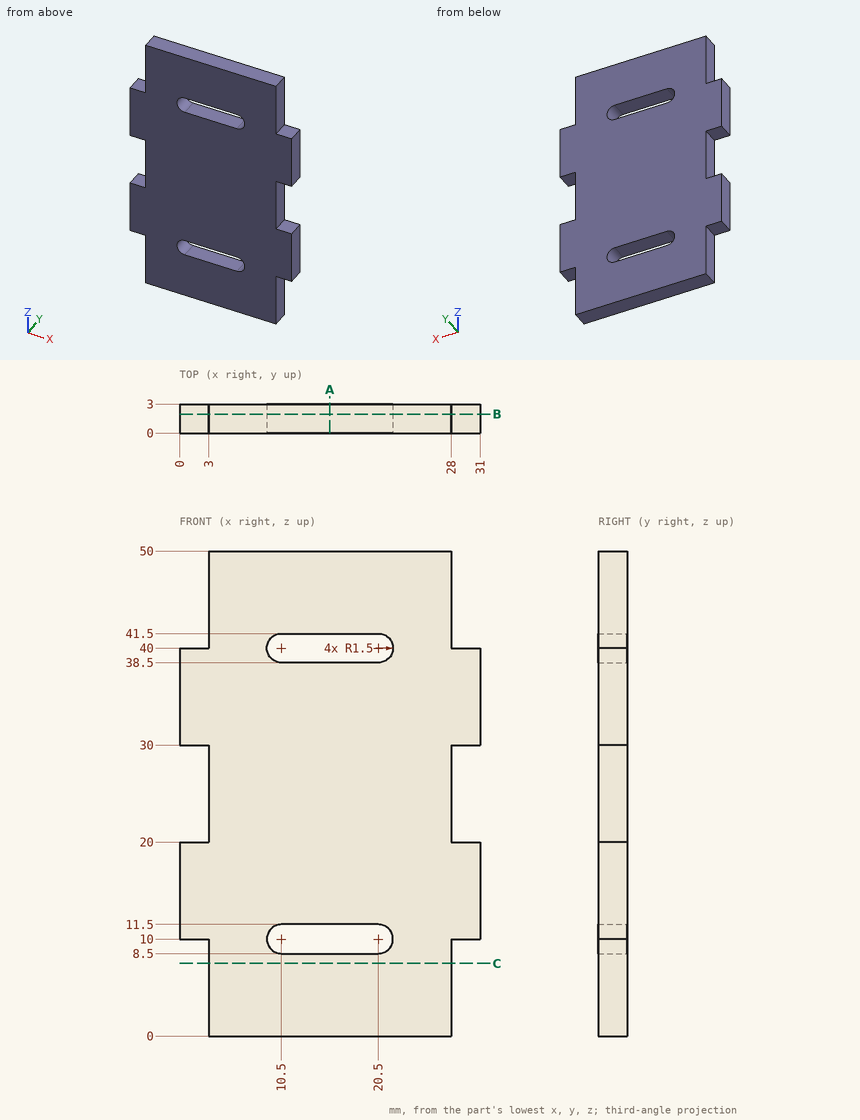
Print and shaded views of the part. All mm, measured from the part's lowest x, y and z. Give positions to 0.01 mm unless a question says otherwise; leave off trailing zeros. Loops run counter-clockwise (first coordinate to the right, second up) from the corner with the lowest first, then second, coordinate; pieces in that order, holes last. Notation, with made-up numbers: (20, -33.5) -> (37, -33.5) arc R7 ccw to (37, -22.5) -> close; hole circle Ø7 at (41, -11.75). An arc over 180 degrees is marked (long way). Use CSV: the item, a comma, the result in double quotes. Start each with the question number.
1) Wall check: line 1 (Z direction, x = 14, y = 0.5); line 2 (Z direction, x = 28.5, y = 1.1); line 3 (Z direction, x = 9.5, y = 1.3). Give the ranges that are in metal, low to high.
2) Slice it at A-A on x = 15.5. Give the cut face in (y, z).
3) Slice it at B-B on y = 1.95. Give the cut face in (x, z).
4) Flat gauge pins, fed straight in: pin 1 Ø0.9 at (x, y) = (30, 1) entering from -Z; pin 2 Ø1.5 at (y, z) = (2, 44) entering from +X; pin 3 Ø0.9 at (y, z) = (1.5, 22.5) entering from -X. Where does each tip first touch, or does it go through?
5) Slice it at C-C on z = 7.5. Give the cut face in (x, y).
Computed values:
1,line 1,"z = 0 to 8.5, 11.5 to 38.5, 41.5 to 50"
1,line 2,"z = 10 to 20, 30 to 40"
1,line 3,"z = 0 to 8.88, 11.12 to 38.88, 41.12 to 50"
2,outline,"(0, 0) -> (3, 0) -> (3, 8.5) -> (0, 8.5) -> close; (0, 11.5) -> (3, 11.5) -> (3, 38.5) -> (0, 38.5) -> close; (0, 41.5) -> (3, 41.5) -> (3, 50) -> (0, 50) -> close"
3,outline,"(0, 10) -> (3, 10) -> (3, 0) -> (28, 0) -> (28, 10) -> (31, 10) -> (31, 20) -> (28, 20) -> (28, 30) -> (31, 30) -> (31, 40) -> (28, 40) -> (28, 50) -> (3, 50) -> (3, 40) -> (0, 40) -> (0, 30) -> (3, 30) -> (3, 20) -> (0, 20) -> close; hole (10.5, 8.5) -> (20.5, 8.5) arc R1.5 ccw to (20.5, 11.5) -> (10.5, 11.5) arc R1.5 ccw to start; hole (10.5, 38.5) -> (20.5, 38.5) arc R1.5 ccw to (20.5, 41.5) -> (10.5, 41.5) arc R1.5 ccw to start"
4,pin 1,"stops at z = 10"
4,pin 2,"stops at x = 28"
4,pin 3,"stops at x = 3"
5,outline,"(3, 0) -> (28, 0) -> (28, 3) -> (3, 3) -> close"
